Answer from the drawing. Dimensions are ordinates in mm from the lowest x, y and z of the part. Round coordinates to 2 decimals unless told otherwise and drop trailing zeros. Order: outer loops, then holes, each group sorted by start corner. A loop starts at its lowest first (then second) coordinate and runs counter-clockwise, first axis right, second up. Notation, with made-up numbers: M -34.75,-30.75 L -2.75,-30.75 A29 ccw -2.75,3.25 Z; hole C -22,62.5 d11. An arc over 180 degrees is marked long. Answer as a JSON object with one key per item and string values. Group by question number.
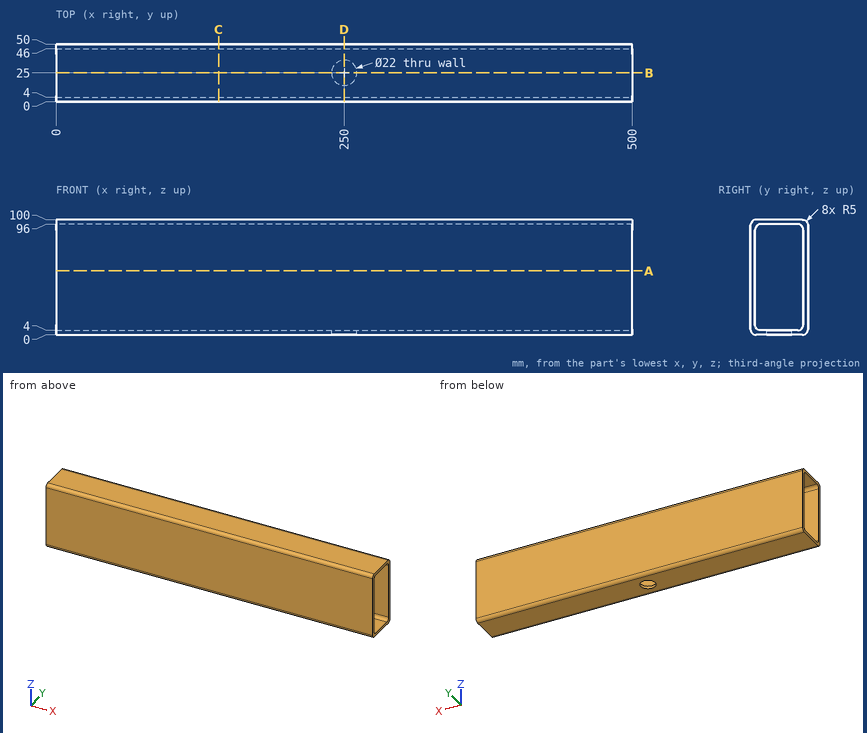
Item 1: Consider L1, parallel to Z at x = 139.5, y = 34; L2, parallel to Y at x = 406, z = 83; L3, parallel to Z at x = 123.5, y = 8. Determine where each line is inside the solid, lowest interval first.
Item 2: Find section D-D (x = 250). Give the vertices of the cut face in (y, z), and give its area (3 significant figures).
Item 3: Find section A-A (z = 55.5). Give the vertices of the cut face in (x, y), and give its area (3 significant figures).
Item 4: Find section B-B (y = 25). Give the vertices of the cut face in (x, z), and give its area (3 significant figures).
Item 5: This flat-tipped pin is pushed along its axis until it touches: pin 1 (13 mm diameter, centred on x = 250, y = 25, fed in from -Z). Where does it stop, or does it pass through?
Item 6: Find section C-C (x = 141). Give the vertices of the cut face in (y, z), and give its area (3 significant figures).
Responses:
{
 "1": {"L1": "z = 0 to 4, 96 to 100", "L2": "y = 0 to 4, 46 to 50", "L3": "z = 0 to 4.1, 95.9 to 100"},
 "2": {"outline": "M 0,5 A5 ccw 5,0 L 14,0 L 14,4 L 9,4 A5 cw 4,9 L 4,91 A5 cw 9,96 L 41,96 A5 cw 46,91 L 46,9 A5 cw 41,4 L 36,4 L 36,0 L 45,0 A5 ccw 50,5 L 50,95 A5 ccw 45,100 L 5,100 A5 ccw 0,95 Z", "area": "1,050 mm^2"},
 "3": {"outline": "M 0,0 L 500,0 L 500,4 L 0,4 Z; M 0,46 L 500,46 L 500,50 L 0,50 Z", "area": "4,000 mm^2"},
 "4": {"outline": "M 0,0 L 239,0 L 239,4 L 0,4 Z; M 0,96 L 500,96 L 500,100 L 0,100 Z; M 261,0 L 500,0 L 500,4 L 261,4 Z", "area": "3,910 mm^2"},
 "5": {"pin 1": "stops at z = 96"},
 "6": {"outline": "M 0,5 A5 ccw 5,0 L 45,0 A5 ccw 50,5 L 50,95 A5 ccw 45,100 L 5,100 A5 ccw 0,95 Z; hole M 4,9 A5 ccw 9,4 L 41,4 A5 ccw 46,9 L 46,91 A5 ccw 41,96 L 9,96 A5 ccw 4,91 Z", "area": "1,140 mm^2"}
}
